```python
from build123d import *

# Parameters (mm, degrees)
BOSS_EXTRUDE1_DEPTH = 29
CUT_EXTRUDE1_START  = 1.5
CUT_EXTRUDE1_DEPTH  = 26


# Read off the part's stored shape, not the designer's step: Cut-Extrude1
with BuildPart() as part:
    # Sketch1 → Boss-Extrude1 (new body)
    with BuildSketch(Plane(origin=(0, 0, 0), x_dir=(0, 0, -1), z_dir=(1, 0, 0))):
        with BuildLine():
            Line((0, 40), (0, 0))
            Line((0, 0), (30, 0))
            add(Edge.make_bspline(
                [(10, 40), (28.045726498, 24.235315383), (30, 0)],
                knots=[0, 0, 0, 1, 1, 1], degree=2))
            Line((10, 40), (0, 40))
        make_face()
    extrude(amount=BOSS_EXTRUDE1_DEPTH)

    # Cut-Extrude1 outline → Cut-Extrude1 (cut)
    with BuildSketch(Plane.YZ.offset(CUT_EXTRUDE1_START)):
        with BuildLine():
            Line((0, 0), (0, -28.5))
            add(Edge.make_bspline(
                [(0, -28.5), (24.235315383, -26.545726498), (40, -8.5)],
                knots=[0, 0, 0, 1, 1, 1], degree=2))
            Line((40, -8.5), (40, 0))
            Line((40, 0), (0, 0))
        make_face()
    extrude(amount=CUT_EXTRUDE1_DEPTH, mode=Mode.SUBTRACT)


solid = part.part
```
Build history of the part. All positions in model axes, mm. A direction names the side the tool comes from. Give positions to 0.01 mm unless a question says otherwise; leave off trailing zeros.
1) Probe line 1 along X through (y, z) = (9, -22); line 2 along Y through (x, z) = (12.75, -14); line 3 along Y through (x, z) = (25.5, -16). List the from-to ranges inside material, lowest first.
Values follow:
line 1: x = 0 to 1.5, 27.5 to 29
line 2: y = 34.59 to 36.2
line 3: y = 32.24 to 34.02
2) Two-plate mould, pull along Z, no slides. Class faces 3 (the face through (28, 20, 0)), 4 (the face through (1.5, 15, -11)): released by +Z, released by -Z, zero draft, split by the parting line, or undercut.
Values follow:
face 3: released by +Z
face 4: zero draft
3) Drop flat-ended pins along their axis: P1, Ø1.5, axis at x = 24.5, z = -15.5, coming from the -Y side; P2, Ø1.5, axis at x = 16, y = 32, coming from the +Z side; P3, Ø12, axis at x = 7.5, y = 31.5, coming from the -Z side. Give the stop position or say it passes through.
Values follow:
P1: stops at y = 31.93
P2: stops at z = -15.58
P3: stops at z = -22.18
4) 3-axis set-ups, long thin cutter, end or side, ignore diameter. For faces 1 (the face through (14, 40, -9)), 2 (the face through (27.5, 15, -11)): which of +Z, -Z, +X, -X, +Y, -Y reach the whole face in a straight line?
Values follow:
face 1: +Z, -Z, +X, -X, +Y
face 2: +Z, -Y
